The listing builds one solid part. Answer for the finished solid, in the listing's coordinates (mm). A direction names the side the tool comes from. Give positions to 0.01 mm unless a question says otherwise; leave off trailing zeros. Write each loop counter-clockwise with the first axis right and the second up, starting at its lowest first coordinate (ties: lowest second). Pieces come first, ordered by that corner, then holes. Notation, with made-up numbers: (-29, 70) -> (16, 70) arc R21 cw to (16, 86) -> close; hole circle Ø6 at (-5, -40). An arc over 180 degrees is marked (long way). One line per question, with ' | ' between items.
from build123d import *

# Parameters (mm, degrees)
F0_W     = 73.406
F0_H     = 28.575
F1_DEPTH = 25.4
F2_W     = 73.406
F2_H     = 28.575
F3_DEPTH = 1.524
F4_W     = 73.406
F4_H     = 28.575
F5_DEPTH = 1.524


with BuildPart() as f1:
    # F0 (on Front) → F1 (new body)
    with BuildSketch(Plane.XZ):
        Polygon((0, 31.75), (0, 0), (104.648, 0), (73.406, 31.75), align=None)
        with BuildLine():
            Line((49.53, 8.636), (14.478, 8.636))
            ThreePointArc((14.478, 8.636), (8.89, 14.224), (14.478, 19.812))
            Line((14.478, 19.812), (49.53, 19.812))
            ThreePointArc((49.53, 19.812), (55.118, 14.224), (49.53, 8.636))
        make_face(mode=Mode.SUBTRACT)
        with Locations((36.703, 46.0375)):
            Rectangle(F0_W, F0_H)
        Polygon((0, 88.9), (0, 60.325), (73.406, 60.325), (104.648, 88.9), align=None)
        with BuildLine():
            Line((49.53, 69.088), (14.478, 69.088))
            ThreePointArc((14.478, 69.088), (8.89, 74.676), (14.478, 80.264))
            Line((14.478, 80.264), (49.53, 80.264))
            ThreePointArc((49.53, 80.264), (55.118, 74.676), (49.53, 69.088))
        make_face(mode=Mode.SUBTRACT)
    extrude(amount=F1_DEPTH)

    # F2 (on face) → F3 (join)
    with BuildSketch(Plane.XZ.offset(25.4)):
        with Locations((36.703, 46.0375)):
            Rectangle(F2_W, F2_H)
    extrude(amount=F3_DEPTH)

    # F4 (on face) → F5 (join)
    with BuildSketch(Plane(origin=(0, 0, 0), x_dir=(-1, 0, 0), z_dir=(0, 1, 0))):
        with Locations((-36.703, 46.0375)):
            Rectangle(F4_W, F4_H)
    extrude(amount=F5_DEPTH)


solid = f1.part
Item 1: Determine the mould class of faces 5 (the face through (32, -13, 19.812)), 6 (the face through (88.808, -12.522, 74.412)), 7 (the face through (0, -13, 44)), 8 (the face through (52, -25.4, 20)) for opening direction X: pulls with the +X half, pulls with the -X half, needs draft (parallel to the pull), parting line crosses it, or undercut.
Answers below:
face 5: undercut | face 6: pulls with the +X half | face 7: pulls with the -X half | face 8: needs draft
Item 2: Find section C-C (z = 16.5). Write down the section's boundary in (x, y), then the cut area to 3 significant figures.
Answers below:
outline: (0, -25.4) -> (9.37, -25.4) -> (9.37, 0) -> (0, 0) -> close; (54.63, -25.4) -> (88.41, -25.4) -> (88.41, 0) -> (54.63, 0) -> close | area: 1,100 mm²
Item 3: Find section A-A (x = 32.5). Write down the section's boundary in (y, z) (3 decimals).
Answers below:
outline: (-26.924, 31.75) -> (-25.4, 31.75) -> (-25.4, 19.812) -> (0, 19.812) -> (0, 31.75) -> (1.524, 31.75) -> (1.524, 60.325) -> (0, 60.325) -> (0, 69.088) -> (-25.4, 69.088) -> (-25.4, 60.325) -> (-26.924, 60.325) -> close; (-25.4, 0) -> (0, 0) -> (0, 8.636) -> (-25.4, 8.636) -> close; (-25.4, 80.264) -> (0, 80.264) -> (0, 88.9) -> (-25.4, 88.9) -> close
Item 4: Find section D-D (z = 44.5). Write down the section's boundary in (x, y), then the cut area to 3 significant figures.
Answers below:
outline: (0, -26.92) -> (73.41, -26.92) -> (73.41, 1.52) -> (0, 1.52) -> close | area: 2,090 mm²
Item 5: A tool of negligible diameter and unlimited length cuts with its end or side. For faces 1 (the face through (52, 0, 81)), 2 (the face through (52, -25.4, 81)), 3 (the face through (52, 0, 20)), 4 (the face through (8.89, -12.52, 74.55)), from which of +Z, -Z, +X, -X, +Y, -Y can it reach the whole face along a straight path? Write none if from no direction.
Answers below:
face 1: +Z, +X, -X, +Y | face 2: +Z, +X, -X, -Y | face 3: -Z, +X, -X, +Y | face 4: +Y, -Y
Item 6: Find section B-B (y = -17.25). Write down the section's boundary in (x, z) (3 decimals).
Answers below:
outline: (0, 0) -> (104.648, 0) -> (73.406, 31.75) -> (73.406, 60.325) -> (104.648, 88.9) -> (0, 88.9) -> close; hole (14.478, 8.636) -> (49.53, 8.636) arc R5.588 ccw to (49.53, 19.812) -> (14.478, 19.812) arc R5.588 ccw to start; hole (14.478, 69.088) -> (49.53, 69.088) arc R5.588 ccw to (49.53, 80.264) -> (14.478, 80.264) arc R5.588 ccw to start
Item 7: Flat-ended cylindrical pins translate along their axes: pin 1 (10 mm diameter, centred on y = -17, z = 59, fed in from +X); pin 2 (0.8 mm diameter, centred on x = 29.5, y = 1, fed in from -Z); pin 3 (9.5 mm diameter, centred on x = 50.5, z = 14.5, fed in from -Y); pin 4 (1 mm diameter, centred on x = 42.5, z = 71, fed in from +Y). Find the tip coordinate at first contact, or state that the pin passes through.
Answers below:
pin 1: x = 77.42 | pin 2: z = 31.75 | pin 3: y = -25.4 | pin 4: through
Item 8: Consider line 1 (Z direction, x = 43, y = -8); line 2 (Z direction, x = 50, y = -1.25); line 3 (Y direction, x = 53, z = 63.5). Determine where each line is inside the solid, lowest interval first. Write a range as [from, to].
Answers below:
line 1: [0, 8.64], [19.81, 69.09], [80.26, 88.9] | line 2: [0, 8.66], [19.79, 69.11], [80.24, 88.9] | line 3: [-25.4, 0]
